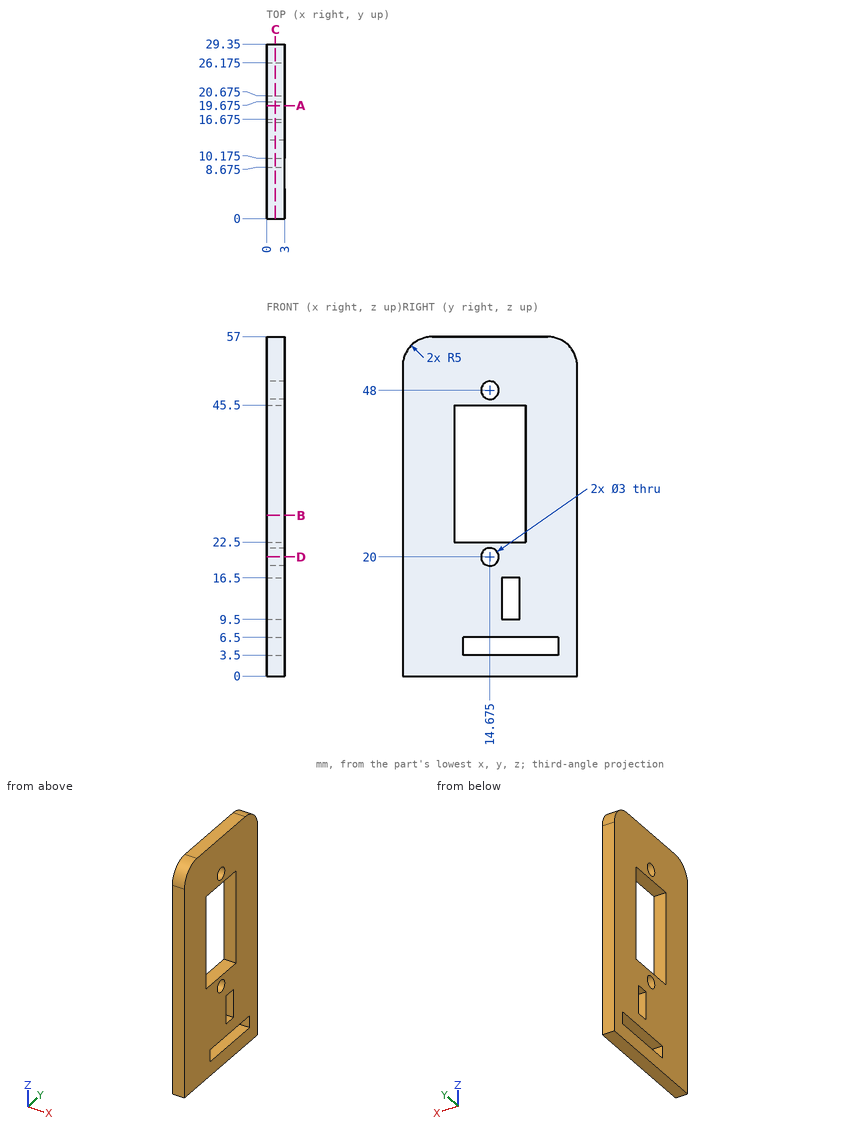
Job drawing, mm, ordinate dimensions from the low corner. One solid piece. Coordinates: 2 decimals unless noted, no trailing zeros. Write each loop counter-clockwise with the first axis right and the second up, starting at its lowest first coordinate (ties: lowest second). Pieces come first, ordered by that corner, then holes. Notation, with made-up numbers: (73.25, -24.5) - (112.25, -24.5) arc R19 ccw to (112.25, -13.5) - close; hole circle Ø8 at (73, 49). An arc over 180 degrees is marked (long way). Use a Markdown table: item, result. Add a question column.
Item 1: Band-saw the part on B-B, the plane z = 27. Give the cut face in (x, y) (3 decimals), and give its area (4 significant figures).
Item 2: Drill centre lines: L1, parallel to Z at x = 2.7, y = 18; L2, parallel to Z at x = 1.3, y = 20; L3, parallel to Z at x = 0.7, y = 21.75. Where is each one in solid material? Low to high. Write a range as from..to.
Item 3: Flat gauge pin, fed straight in: pin 1 (2.5 mm diameter, centred on y = 14.675, z = 20, fed in from +X). Where does the tip first touch, or does it go through?
Item 4: Band-saw the part on D-D, the plane z = 20. Give the cut face in (x, y) (3 decimals).
Item 5: Band-saw the part on A-A, the plane y = 19. Give the cut face in (x, z).
Item 6: Band-saw the part on C-C, the plane x = 1.45. Give the cut face in (y, z) (3 decimals).
Numbers:
| question | item | result |
|---|---|---|
| 1 | outline | (0, 0) - (3, 0) - (3, 8.675) - (0, 8.675) - close; (0, 20.675) - (3, 20.675) - (3, 29.35) - (0, 29.35) - close |
| 1 | area | 52.05 mm2 |
| 2 | L1 | 0..3.5, 6.5..9.5, 16.5..22.5, 45.5..57 |
| 2 | L2 | 0..3.5, 6.5..22.5, 45.5..57 |
| 2 | L3 | 0..3.5, 6.5..57 |
| 3 | pin 1 | through |
| 4 | outline | (0, 0) - (3, 0) - (3, 13.175) - (0, 13.175) - close; (0, 16.175) - (3, 16.175) - (3, 29.35) - (0, 29.35) - close |
| 5 | outline | (0, 0) - (3, 0) - (3, 3.5) - (0, 3.5) - close; (0, 6.5) - (3, 6.5) - (3, 9.5) - (0, 9.5) - close; (0, 16.5) - (3, 16.5) - (3, 22.5) - (0, 22.5) - close; (0, 45.5) - (3, 45.5) - (3, 57) - (0, 57) - close |
| 6 | outline | (0, 0) - (29.35, 0) - (29.35, 52) arc R5 ccw to (24.35, 57) - (5, 57) arc R5 ccw to (0, 52) - close; hole (8.675, 22.5) - (20.675, 22.5) - (20.675, 45.5) - (8.675, 45.5) - close; hole (10.175, 3.5) - (26.175, 3.5) - (26.175, 6.5) - (10.175, 6.5) - close; hole circle Ø3 at (14.675, 20); hole circle Ø3 at (14.675, 48); hole (16.675, 9.5) - (19.675, 9.5) - (19.675, 16.5) - (16.675, 16.5) - close |
